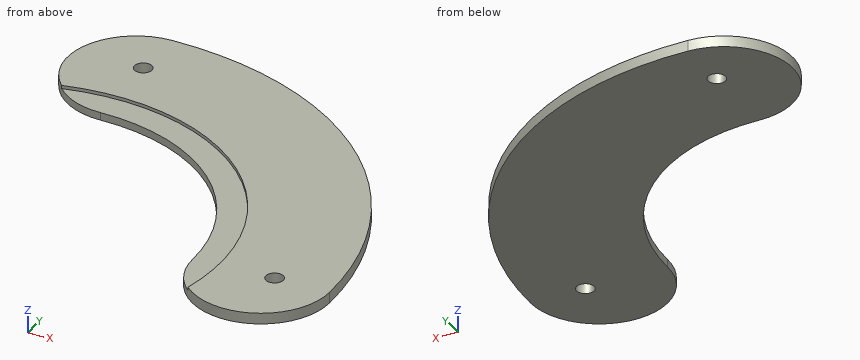
```python
from build123d import *

# Parameters (mm, degrees)
SKETCH_R     = 1.6
PAD_DEPTH    = 2
SKETCH001_R  = 40
POCKET_DEPTH = 0.6


with BuildPart() as part:
    # Sketch → Pad (new body)
    with BuildSketch(Plane.XY):
        with BuildLine():
            ThreePointArc((35, -7.3e-05), (24.748759, 24.748716), (-1.3e-05, 35))
            ThreePointArc((0, 60), (-12.5, 47.500006), (-1.3e-05, 35))
            ThreePointArc((60, -0.000125), (42.426451, 42.426363), (0, 60))
            ThreePointArc((35, -7.3e-05), (47.499974, -12.500099), (60, -0.000125))
        make_face()
        with Locations((50, -0.000104)):
            Circle(SKETCH_R, mode=Mode.SUBTRACT)
        with Locations((-1.8e-05, 50)):
            Circle(SKETCH_R, mode=Mode.SUBTRACT)
    extrude(amount=PAD_DEPTH)

    # Sketch001 (on Face8 of Pad) → Pocket (cut)
    with BuildSketch(Plane.XY.offset(2)):
        Circle(SKETCH001_R)
    extrude(amount=-POCKET_DEPTH, mode=Mode.SUBTRACT)


solid = part.part
```
Work out the finished part from the listing and answer in its coordinate system (mm). Give positions to 0.01 mm unless a question says otherwise; leave off trailing zeros. Loops run counter-clockwise (first coordinate to the right, second up) from the corner with the lowest first, then second, coordinate; pieces in that order, holes last. Notation, with made-up numbers: M 77,26 L 85,26 A28 ccw 85,61 Z; hole C -7,56.25 d1. An arc over 180 degrees is marked long. One line per item, written item: value. Start each with the question number.
1. This flat-tipped pin is pushed along its axis until it touches: P1, Ø3, axis at x = 24, y = 25.5, coming from the +Z side. Where does it stop, or does it pass through?
2. Find the intervals of material crossed by probe 1 along Y at (x, z) = (51, 1.2); probe 2 along Y at (x, z) = (50, 1.05); probe 3 along X at (y, z) = (2.5, 0.5), in increasing order.
3. Find section D-D (z = 0.6). Give the vertices of the cut face in (x, y).
4. Find section A-A (x = 50). Give the vertices of the cut face in (y, z).
5. Find section C-C (x = 31.5). Give the vertices of the cut face in (y, z).
Reported:
1. P1: stops at z = 1.4
2. probe 1: y = -12 to -1.25, 1.25 to 31.61
2. probe 2: y = -12.25 to -1.6, 1.6 to 33.17
2. probe 3: x = 34.91 to 59.95
3. outline: M 0,35 A35 cw 35,0 A12.5 ccw 60,0 A60 ccw 0,60 A12.5 ccw Z; hole C 0,50 d3.2; hole C 50,0 d3.2
4. outline: M -12.25,0 L -1.6,0 L -1.6,2 L -12.25,2 Z; M 1.6,0 L 33.17,0 L 33.17,2 L 1.6,2 Z
5. outline: M 15.26,0 L 51.07,0 L 51.07,2 L 24.65,2 L 24.65,1.4 L 15.26,1.4 Z
